CAD build for the part. Positions are in the model's coordinates, mm. A direction names the side the tool comes from. Coordinates: 2 decimals unless noted, no trailing zeros. Loops run counter-clockwise (first coordinate to the right, second up) from the corner with the lowest first, then second, coordinate; pieces in that order, holes last. Notation, with made-up numbers: (-16.75, -8.5) -> (11.25, -8.5) arc R24 ccw to (11.25, 29.5) -> close; hole circle Ø1 at (48, 15). An arc over 180 degrees is marked (long way). Write each question's results on one line, items separated by ' | '.
```python
from build123d import *

# Parameters (mm, degrees)
SKETCH1_W           = 35.35
SKETCH1_H           = 47.35
SKETCH1_W_2         = 10
SKETCH1_H_2         = 24
BOSS_EXTRUDE1_DEPTH = 3.175
SKETCH2_W           = 3.175
SKETCH2_H           = 10
SKETCH2_W_2         = 1.5875
SKETCH2_W_3         = 7.5
SKETCH2_H_2         = 3.175
CUT_EXTRUDE1_DEPTH  = 4.175


with BuildPart() as part:
    # Sketch1 → Boss-Extrude1 (new body)
    with BuildSketch(Plane(origin=(0, 0, 0), x_dir=(0, 0, -1), z_dir=(1, 0, 0))):
        with Locations((17.675, 23.675)):
            Rectangle(SKETCH1_W, SKETCH1_H)
        with Locations((20.175, 18.175)):
            Rectangle(SKETCH1_W_2, SKETCH1_H_2, mode=Mode.SUBTRACT)
    extrude(amount=BOSS_EXTRUDE1_DEPTH)

    # Sketch2 → Cut-Extrude1 (cut, through all)
    with BuildSketch(Plane(origin=(3.175, 0, 0), x_dir=(0, 0, -1), z_dir=(1, 0, 0))):
        with Locations((33.7625, 33.675)):
            Rectangle(SKETCH2_W, SKETCH2_H)
        with Locations((33.7625, 13.675)):
            Rectangle(SKETCH2_W, SKETCH2_H)
        with Locations((9.0875, 13.675)):
            Rectangle(SKETCH2_W, SKETCH2_H)
        with Locations((9.0875, 33.675)):
            Rectangle(SKETCH2_W, SKETCH2_H)
        with Locations((0.79375, 33.675)):
            Rectangle(SKETCH2_W_2, SKETCH2_H)
        with Locations((0.79375, 13.675)):
            Rectangle(SKETCH2_W_2, SKETCH2_H)
        with Locations((24.1, 45.7625)):
            Rectangle(SKETCH2_W_3, SKETCH2_H_2)
        with Locations((9.1, 45.7625)):
            Rectangle(SKETCH2_W_3, SKETCH2_H_2)
        with Locations((9.1, 1.5875)):
            Rectangle(SKETCH2_W_3, SKETCH2_H_2)
        with Locations((24.1, 1.5875)):
            Rectangle(SKETCH2_W_3, SKETCH2_H_2)
    extrude(amount=-CUT_EXTRUDE1_DEPTH, mode=Mode.SUBTRACT)


solid = part.part
```
Q1. Cut at A-A on z = -21.5. Write the cut outline in (x, y) (3 decimals), and give its area (3 significant figures).
Results are:
outline: (0, 3.175) -> (3.175, 3.175) -> (3.175, 6.175) -> (0, 6.175) -> close; (0, 30.175) -> (3.175, 30.175) -> (3.175, 44.175) -> (0, 44.175) -> close | area: 54.0 mm^2
Q2. Cut at B-B on y = 7. Write the cut outline in (x, z) (3 decimals), and give its area (3 significant figures).
Results are:
outline: (0, -35.35) -> (3.175, -35.35) -> (3.175, -25.175) -> (0, -25.175) -> close; (0, -15.175) -> (3.175, -15.175) -> (3.175, 0) -> (0, 0) -> close | area: 80.5 mm^2
Q3. Which spindle directions (+Z, -Z, +X, -X, +Y, -Y) get a long thin tool onto all of the face, cutting with end or side? Do faces 4 (the flat face through (2, 46, -5.35)), 5 (the flat face through (2, 14, -1.588)), 6 (the flat face through (2, 2, -12.85)). Say none if no direction does.
Results are:
face 4: +X, -X, +Y | face 5: +Z, +X, -X | face 6: +X, -X, -Y
Q4. Drop a flat-ended pin along its axis: pin 1 (1.6 mm diameter, centred on x = 2, y = 14.5, fed in from +Z). Give the stop position or say it passes through.
Results are:
pin 1: z = -1.59
Q5. Pull direction Y, two halves, no side cores. Call faces 1 (the flat face through (2, 3.175, -9)), 2 (the flat face through (2, 30.175, -20)), 3 (the flat face through (2, 46, -12.85)): +Y half, -Y half, draft (parallel to the pull), parting line (faces both ways), or undercut.
Results are:
face 1: -Y half | face 2: undercut | face 3: draft
Q6. Cut at C-C on z = -8. Write the cut outline in (x, y) (3 decimals).
Results are:
outline: (0, 3.175) -> (3.175, 3.175) -> (3.175, 8.675) -> (0, 8.675) -> close; (0, 18.675) -> (3.175, 18.675) -> (3.175, 28.675) -> (0, 28.675) -> close; (0, 38.675) -> (3.175, 38.675) -> (3.175, 44.175) -> (0, 44.175) -> close
Q7. Wall check: L1, parallel to Y at x = 0.8, z = -10 (3 decimals); L2, parallel to Z at x = 1.35, y = 37 (1 decimal); L3, parallel to Z at x = 2.15, y = 26.5 (3 decimals). Give the ranges that are in metal, low to high. Write a range as from..to.
Results are:
L1: 3.175..8.675, 18.675..28.675, 38.675..44.175 | L2: -32.2..-10.7, -7.5..-1.6 | L3: -35.35..-25.175, -15.175..0
Q8. Cut at D-D on x = 0.7. Give the number of separate pieces and of enclosed holes in the cut face, and give its area (3 significant figures).
Results are:
separate pieces: 1 | enclosed holes: 3 | area: 1,180 mm^2
